Model file for the job. Use its own axes, mm. A direction names the side the tool comes from. Coordinates: 2 decimals unless noted, no trailing zeros. Loops run counter-clockwise (first coordinate to the right, second up) from the corner with the lowest first, then second, coordinate; pieces in that order, holes last.
from build123d import *

# Parameters (mm, degrees)
SKETCH1_R                = 18
SKETCH1_R_2              = 7
BOSS_EXTRUDE1_DEPTH      = 4
BOSS_EXTRUDE2_DEPTH      = 30
SKETCH3_R                = 18
SKETCH3_R_2              = 12.5
BOSS_EXTRUDE3_DEPTH      = 1
BOSS_EXTRUDE3_DEPTH_BACK = 3


with BuildPart() as part:
    # Sketch1 → Boss-Extrude1 (new body)
    with BuildSketch(Plane(origin=(0, 0, 0), x_dir=(1, 0, 0), z_dir=(0, 1, 0))):
        Circle(SKETCH1_R)
        Circle(SKETCH1_R_2, mode=Mode.SUBTRACT)
    extrude(amount=BOSS_EXTRUDE1_DEPTH)

    # Sketch2 → Boss-Extrude2 (add)
    with BuildSketch(Plane.XZ):
        with BuildLine():
            Line((4.732447, 11.569526), (7.5, 16.363068))
            ThreePointArc((7.5, 16.363068), (0, 18), (-7.5, 16.363068))
            Line((-7.5, 16.363068), (-4.732447, 11.569526))
            ThreePointArc((-4.732447, 11.569526), (0, 12.5), (4.732447, 11.569526))
        make_face()
        with BuildLine():
            Line((11.569526, -4.732447), (16.363068, -7.5))
            ThreePointArc((16.363068, -7.5), (18, 0), (16.363068, 7.5))
            Line((16.363068, 7.5), (11.569526, 4.732447))
            ThreePointArc((11.569526, 4.732447), (12.5, 0), (11.569526, -4.732447))
        make_face()
        with BuildLine():
            Line((-4.732447, -11.569526), (-7.5, -16.363068))
            ThreePointArc((-7.5, -16.363068), (0, -18), (7.5, -16.363068))
            Line((7.5, -16.363068), (4.732447, -11.569526))
            ThreePointArc((4.732447, -11.569526), (0, -12.5), (-4.732447, -11.569526))
        make_face()
        with BuildLine():
            Line((-11.569526, 4.732447), (-16.363068, 7.5))
            ThreePointArc((-16.363068, 7.5), (-18, 0), (-16.363068, -7.5))
            Line((-16.363068, -7.5), (-11.569526, -4.732447))
            ThreePointArc((-11.569526, -4.732447), (-12.5, 0), (-11.569526, 4.732447))
        make_face()
    extrude(amount=BOSS_EXTRUDE2_DEPTH)

    # Sketch3 → Boss-Extrude3 (add, two sides)
    with BuildSketch(Plane.XZ.offset(30)) as boss_extrude3_sk:
        Circle(SKETCH3_R)
        Circle(SKETCH3_R_2, mode=Mode.SUBTRACT)
    extrude(amount=BOSS_EXTRUDE3_DEPTH)
    extrude(boss_extrude3_sk.sketch, amount=-BOSS_EXTRUDE3_DEPTH_BACK)


solid = part.part
Q1. Slice it at C-C (x = 10.5). List the corners of the cut face in (y, z).
Answers:
outline: (-31, -14.62) - (-27, -14.62) - (-27, -6.78) - (-31, -6.78) - close; (-31, 6.78) - (-27, 6.78) - (-27, 14.62) - (-31, 14.62) - close; (0, -14.62) - (4, -14.62) - (4, 14.62) - (0, 14.62) - close
Q2. Slice it at A-A (z = 0). List the corners of the cut face in (x, y).
Answers:
outline: (-18, -31) - (-12.5, -31) - (-12.5, 0) - (-7, 0) - (-7, 4) - (-18, 4) - close; (7, 0) - (12.5, 0) - (12.5, -31) - (18, -31) - (18, 4) - (7, 4) - close
Q3. Slice it at B-B (y = -18.5). List the corners of the cut face in (x, z).
Answers:
outline: (-16.36, -7.5) - (-11.57, -4.73) arc R12.5 cw to (-11.57, 4.73) - (-16.36, 7.5) arc R18 ccw to start; (-7.5, -16.36) arc R18 ccw to (7.5, -16.36) - (4.73, -11.57) arc R12.5 cw to (-4.73, -11.57) - close; (-7.5, 16.36) - (-4.73, 11.57) arc R12.5 cw to (4.73, 11.57) - (7.5, 16.36) arc R18 ccw to start; (11.57, -4.73) - (16.36, -7.5) arc R18 ccw to (16.36, 7.5) - (11.57, 4.73) arc R12.5 cw to start
Q4. Which spindle directions (+Z, -Z, +X, -X, +Y, -Y) get a long thin tool onto all of the face, cutting with end or side? Do faces 5 (the flat face through (6.097, -14.79, 13.933)), 6 (the flat face through (14, -14.79, 6.136)), 7 (the flat face through (-6.097, -14.79, -13.933)), 8 (the flat face through (-14, -14.79, -6.136)). Say none if no direction does.
Answers:
face 5: +X
face 6: +Z
face 7: -X
face 8: -Z
Q5. Mould opens along Z. For faces 1 (the flat face through (-11, -27, 11)), 2 (the flat face through (7, 0, 3)), 3 (the flat face through (-13.933, -14.79, 6.097)), 4 (the flat face through (13.933, -14.79, -6.097)) say: +Z half, -Z half, draft (parallel to the pull), parting line (faces both ways), or undercut.
Answers:
face 1: undercut
face 2: undercut
face 3: +Z half
face 4: -Z half
Q6. Drill centre lines: line 1 (Y direction, x = 11.5, z = -7.5); line 2 (Z direction, x = 0, y = -30); line 3 (X direction, y = 2.45, z = 0). Where is each one in solid material? Low to high.
Answers:
line 1: y = -31 to -27, 0 to 4
line 2: z = -18 to -12.5, 12.5 to 18
line 3: x = -18 to -7, 7 to 18
Q7. Flat gauge pins, fed straight in: P1, Ø12, axis at x = -3, z = -8.5, coming from the -Y side; P2, Ø1.5, axis at y = -1.5, z = 8.5, coming from the -X side; P3, Ø4, axis at y = -13.5, z = -14, coming from the -X side; P4, Ø10, axis at x = 7, z = -2, coming from the -Y side. Where does each tip first touch, or does it go through?
Answers:
P1: stops at y = -31
P2: passes through
P3: stops at x = -7.29
P4: stops at y = 0
Q8. Slice it at D-D (z = -9). List the corners of the cut face in (x, y), and give its area (3 significant figures).
Answers:
outline: (-15.59, -31) - (-8.67, -31) - (-8.67, -27) - (-15.59, -27) - close; (-15.59, 0) - (15.59, 0) - (15.59, 4) - (-15.59, 4) - close; (8.67, -31) - (15.59, -31) - (15.59, -27) - (8.67, -27) - close
area: 180 mm2
